The listing builds one solid part. Answer for the finished solid, in the listing's coordinates (mm). Give positions to 0.01 mm unless a question says otherwise; leave off trailing zeros. Write each loop counter-clockwise with the first axis right and the second up, starting at its lowest first coordinate (ties: lowest second). Pieces come first, ordered by that corner, then holes. Notation, with made-up numbers: (-4, 88.25) - (32, 88.25) arc R30 ccw to (32, 116.25) - close; hole circle Ø9 at (15, -29.5). An arc over 180 degrees is marked (long way). Answer as CSV lines item,"result". Start each with the question number.
(1) Find section C-C (y = -18). Write down the section's boundary in (x, z).
(2) Find section A-A (z = 1.4). Write down the section's boundary in (x, y), then the cut area to 3 significant figures.
(3) Find section D-D (x = 9.75). Write down the section's boundary in (y, z).
(4) Straight lines are drawn through the part: probe 1 along Y at (x, z) = (4, 0.95); probe 2 along X at (y, z) = (10.5, 1.8); probe 3 along Y at (x, z) = (-8.75, 1). For each, find the intervals that lie inside material, in ascending order.
(5) Find section B-B (y = 16). Write down the section's boundary in (x, z), then the cut area to 3 significant figures.
(6) For a pull along Y with two mould halves and no side action, classify faces 1 (the face through (3, -24.048, 1)), 2 (the face through (1.824, -18.98, 1.521)), 3 (the face through (3.17, 16.49, 1.52)), 4 (the face through (10.907, 17.417, 1.479)) as pulls with the +Y half, pulls with the -Y half, needs draft (parallel to the pull), parting line crosses it, or undercut.
from build123d import *

# Parameters (mm, degrees)
SKETCH1_W           = 25
SKETCH1_H           = 44
BOSS_EXTRUDE1_DEPTH = 3
CHAMFER1_SIZE       = 10
CHAMFER2_SIZE       = 5
SKETCH2_R           = 1.55
CUT_EXTRUDE1_DEPTH  = 3


with BuildPart() as part:
    # Sketch1 → Boss-Extrude1 (new body)
    with BuildSketch(Plane.XY):
        with Locations((0.872372372, -2.048048048)):
            Rectangle(SKETCH1_W, SKETCH1_H)
    extrude(amount=BOSS_EXTRUDE1_DEPTH)

    # Chamfer1
    chamfer1_edges = [part.edges().sort_by_distance(p)[0] for p in [
        (-11.627627628, 19.951951952, 1.5),
        (-11.627627628, -24.048048048, 1.5),
    ]]
    chamfer(chamfer1_edges, length=CHAMFER1_SIZE)

    # Chamfer2
    chamfer2_edges = [part.edges().sort_by_distance(p)[0] for p in [
        (13.372372372, 19.951951952, 1.5),
        (13.372372372, -24.048048048, 1.5),
    ]]
    chamfer(chamfer2_edges, length=CHAMFER2_SIZE)

    # Sketch2 → Cut-Extrude1 (cut)
    with BuildSketch(Plane.XY.offset(3)):
        with Locations((3.372372372, 14.951951952)):
            Circle(SKETCH2_R)
        with Locations((3.372372372, -19.048048048)):
            Circle(SKETCH2_R)
    extrude(amount=-CUT_EXTRUDE1_DEPTH, mode=Mode.SUBTRACT)


solid = part.part
Result set:
1,outline,"(-7.68, 0) - (2.23, 0) - (2.23, 3) - (-7.68, 3) - close; (4.51, 0) - (13.37, 0) - (13.37, 3) - (4.51, 3) - close"
2,outline,"(-11.63, -14.05) - (-1.63, -24.05) - (8.37, -24.05) - (13.37, -19.05) - (13.37, 14.95) - (8.37, 19.95) - (-1.63, 19.95) - (-11.63, 9.95) - close; hole circle Ø3.1 at (3.37, -19.05); hole circle Ø3.1 at (3.37, 14.95)"
2,area,"960 mm^2"
3,outline,"(-22.67, 0) - (18.57, 0) - (18.57, 3) - (-22.67, 3) - close"
4,probe 1,"-24.05 to -20.47, -17.63 to 13.53, 16.37 to 19.95"
4,probe 2,"-11.08 to 13.37"
4,probe 3,"-16.93 to 12.83"
5,outline,"(-5.58, 0) - (2.23, 0) - (2.23, 3) - (-5.58, 3) - close; (4.51, 0) - (12.32, 0) - (12.32, 3) - (4.51, 3) - close"
5,area,"46.9 mm^2"
6,face 1,"pulls with the -Y half"
6,face 2,"undercut"
6,face 3,"undercut"
6,face 4,"pulls with the +Y half"
